from build123d import *

# Parameters (mm, degrees)
ESBO_O1_W                = 450
ESBO_O1_H                = 400
ESBO_O1_W_2              = 440
ESBO_O1_H_2              = 390
RESSALTO_EXTRUS_O1_DEPTH = 450
ESBO_O2_R                = 2.5
RESSALTO_EXTRUS_O2_DEPTH = 183.55
ESBO_O2_3_R              = 2.5
RESSALTO_EXTRUS_O3_DEPTH = 188.55
ESBO_O2_4_R              = 7.5
RESSALTO_EXTRUS_O4_DEPTH = 181.55
ESBO_O3_R                = 2.5
RESSALTO_EXTRUS_O5_DEPTH = 183.45
ESBO_O3_3_R              = 2.5
RESSALTO_EXTRUS_O6_DEPTH = 183.45
RESSALTO_EXTRUS_O7_START = -120.45
ESBO_O3_4_R              = 7.5
RESSALTO_EXTRUS_O7_DEPTH = 120.45


with BuildPart() as part:
    # Esbo_o1 → Ressalto-extrus_o1 (new body)
    with BuildSketch(Plane(origin=(0, 0, 0), x_dir=(0, 0, -1), z_dir=(1, 0, 0))):
        with Locations((225, 200)):
            Rectangle(ESBO_O1_W, ESBO_O1_H)
        with Locations((225, 200)):
            Rectangle(ESBO_O1_W_2, ESBO_O1_H_2, mode=Mode.SUBTRACT)
    extrude(amount=RESSALTO_EXTRUS_O1_DEPTH)

    # Esbo_o2 → Ressalto-extrus_o2 (add)
    with BuildSketch(Plane.XY):
        with Locations((400.68, 282.17)):
            Circle(ESBO_O2_R)
    extrude(amount=-RESSALTO_EXTRUS_O2_DEPTH)

    # Esbo_o2_3 → Ressalto-extrus_o3 (add)
    with BuildSketch(Plane.XY):
        with Locations((347.87, 268.16)):
            Circle(ESBO_O2_3_R)
    extrude(amount=-RESSALTO_EXTRUS_O3_DEPTH)

    # Esbo_o2_4 → Ressalto-extrus_o4 (add)
    with BuildSketch(Plane.XY):
        with Locations((150.03, 199.95)):
            Circle(ESBO_O2_4_R)
    extrude(amount=-RESSALTO_EXTRUS_O4_DEPTH)

    # Esbo_o3 → Ressalto-extrus_o5 (add)
    with BuildSketch(Plane(origin=(0, 0, -450), x_dir=(-1, 0, 0), z_dir=(0, 0, -1))):
        with Locations((-427.35, 285.92)):
            Circle(ESBO_O3_R)
    extrude(amount=-RESSALTO_EXTRUS_O5_DEPTH)

    # Esbo_o3_3 → Ressalto-extrus_o6 (add)
    with BuildSketch(Plane(origin=(0, 0, -450), x_dir=(-1, 0, 0), z_dir=(0, 0, -1))):
        with Locations((-353.49, 348.09)):
            Circle(ESBO_O3_3_R)
    extrude(amount=-RESSALTO_EXTRUS_O6_DEPTH)

    # Esbo_o3_4 → Ressalto-extrus_o7 (add)
    with BuildSketch(Plane(origin=(0, 0, -450), x_dir=(-1, 0, 0), z_dir=(0, 0, -1)).offset(RESSALTO_EXTRUS_O7_START)):
        with Locations(Location((-150.03, 199.95, 0), (0, 0, 180))):
            Circle(ESBO_O3_4_R)
    extrude(amount=RESSALTO_EXTRUS_O7_DEPTH)


solid = part.part
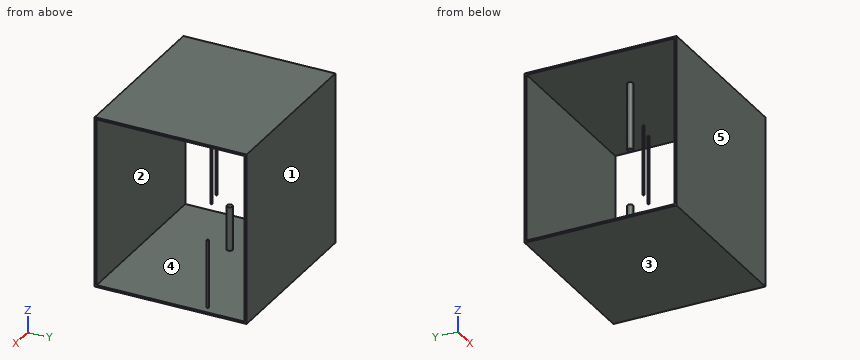
CAD build for the part. Positions are in the model's coordinates, mm. Face numbers are marked on the shaded views. A direction names the side the tool comes from. Give positions to 0.01 mm unless a question says otherwise; leave off trailing zeros. Order: outer loops, then holes, each group sorted by start corner. A loop starts at its lowest first (then second) coordinate and runs counter-clockwise, first axis right, second up. Notation, with made-up numbers: (21.5, 7) - (46.5, 7) arc R20 ccw to (46.5, 18) - close; hole circle Ø11 at (78, 24.5). An arc over 180 degrees is marked (long way). Write each question's results on one line, items separated by ' | '.
1. Saw through at A-A on y = 234.5. List the corners of the cut face in (x, z), and give its area (3 significant figures).
Calculated:
outline: (0, -450) - (450, -450) - (450, -445) - (0, -445) - close; (0, -5) - (450, -5) - (450, 0) - (0, 0) - close | area: 4,500 mm2
2. Pull direction Y, two halves, no side cores. Call the marked faces 3, 4 and 5: released by +Y, released by -Y, zero draft, split by the parting line, or undercut.
Calculated:
face 3: zero draft | face 4: undercut | face 5: released by -Y
3. 3-axis set-ups, long thin cutter, end or side, ignore diameter. For the marked faces 1 and 2: which of +Z, -Z, +X, -X, +Y, -Y reach the whole face in a straight line?
Calculated:
face 1: +Z, -Z, +X, -X, +Y | face 2: +X, -X
4. Saw through at C-C on x = 150.03. List the corners of the cut face in (y, z).
Calculated:
outline: (0, -450) - (400, -450) - (400, 0) - (0, 0) - close; hole (5, -445) - (192.45, -445) - (192.45, -329.55) - (207.45, -329.55) - (207.45, -445) - (395, -445) - (395, -5) - (207.45, -5) - (207.45, -181.55) - (192.45, -181.55) - (192.45, -5) - (5, -5) - close
5. Saw through at B-B on z = -391.5. List the corners of the cut face in (x, y).
Calculated:
outline: (0, 0) - (450, 0) - (450, 5) - (0, 5) - close; (0, 395) - (450, 395) - (450, 400) - (0, 400) - close; circle Ø15 at (150.03, 199.95); circle Ø5 at (353.49, 348.09); circle Ø5 at (427.35, 285.92)
6. Probe L1, parallel to Y at x = 122.5, z = -206.5; L2, parallel to Z at x = 276, y = 83; L3, parallel to Y at x = 401, z = -49. List the from-to ranges inside material, lowest first. Write a range as from..to.
Calculated:
L1: y = 0..5, 395..400 | L2: z = -450..-445, -5..0 | L3: y = 0..5, 279.69..284.65, 395..400
